Part model, mm, in its own coordinate system. A direction names the side the tool comes from. Round coordinates to 2 decimals unless told otherwise and drop trailing zeros. Write each loop counter-clockwise with the first axis right and the second up, starting at its lowest first coordinate (ties: lowest second). Pieces come first, ordered by that corner, then holes. Notation, with made-up numbers: M -16.5,19 L 34.5,19 A18 cw 34.5,47 Z; hole C 58.25,29 d6. An arc over 180 degrees is marked long. Use a Markdown table: item, result. Add a question column.
1) Drop flat-ended pins along their axis: P1, Ø6, axis at x = 1348.5, y = 740, coming from the -Z side; P2, Ø5, axis at x = 292.5, y = 429, coming from the +Z side; P3, Ø10, axis at y = 860, z = -823.5, coming from the +X side. Give the stop position or say it passes through.
2) Slice it at A-A on y = 587. Write the cut outline in (x, z), plus the area to 3 significant figures.
3) Which spindle directions (+Z, -Z, +X, -X, +Y, -Y) get a long thin tool onto all of the face, cutting with end or side? Do faces 4 (the face through (1266, 508, -129)), 5 (the face through (1270, 501, -758)), 6 (the face through (1016, 561, -307)). Say none if no direction does.
4) Slice it at B-B on x = 1042.5. Write the cut outline in (y, z).
5) Slice it at D-D on y = 353. Write the cut outline in (x, z).
6) Slice it at C-C on z = -487.5. Write the cut outline in (x, y).
7) Wall check: probe 1 along Y at (x, z) = (1159, -176); probe 2 along Z at (x, y) = (1097, 419); probe 3 along Z at (x, y) = (921, 594.5). Give the ranges that are in metal, low to high.
8) Two-plate mould, pull along Y, no slides. Class faces 1 (the face through (1524, 376, -258)), 2 (the face through (1274, 762, -258)), 3 (the face through (582, 254, -258)): released by +Y, released by -Y, zero draft, split by the parting line, or undercut.
```python
from build123d import *

# Parameters (mm, degrees)
SKETCH1_W           = 1016
SKETCH1_H           = 508
BOSS_EXTRUDE1_DEPTH = 254
BOSS_EXTRUDE2_DEPTH = 1016
BOSS_EXTRUDE3_DEPTH = 762
SKETCH2_W           = 254
SKETCH2_H           = 254
CUT_EXTRUDE3_DEPTH  = 508


with BuildPart() as part:
    # Sketch1 → Boss-Extrude1 (new body)
    with BuildSketch(Plane(origin=(0, 0, 0), x_dir=(1, 0, 0), z_dir=(0, 1, 0))):
        with Locations((508, 254)):
            Rectangle(SKETCH1_W, SKETCH1_H)
    extrude(amount=BOSS_EXTRUDE1_DEPTH)

    # Sketch1_3 → Boss-Extrude2 (add)
    with BuildSketch(Plane(origin=(0, 0, 0), x_dir=(1, 0, 0), z_dir=(0, 1, 0))):
        Polygon((0, 1016), (0, 508), (1016, 508), (1270, 508), (1270, 1016), align=None)
    extrude(amount=BOSS_EXTRUDE2_DEPTH)

    # Sketch1_4 → Boss-Extrude3 (add)
    with BuildSketch(Plane(origin=(0, 0, 0), x_dir=(1, 0, 0), z_dir=(0, 1, 0))):
        Polygon((1016, 508), (1270, 508), (1524, 508), (1524, 0), (1016, 0), align=None)
    extrude(amount=BOSS_EXTRUDE3_DEPTH)

    # Sketch2 → Cut-Extrude3 (cut)
    with BuildSketch(Plane.ZY.offset(-1016)):
        with Locations((-127, 381)):
            Rectangle(SKETCH2_W, SKETCH2_H)
    extrude(amount=-CUT_EXTRUDE3_DEPTH, mode=Mode.SUBTRACT)


solid = part.part
```
Entries:
| question | item | result |
|---|---|---|
| 1 | P1 | stops at z = -508 |
| 1 | P2 | stops at z = -508 |
| 1 | P3 | stops at x = 1270 |
| 2 | outline | M 0,-1016 L 1270,-1016 L 1270,-508 L 1524,-508 L 1524,0 L 1016,0 L 1016,-508 L 0,-508 Z |
| 2 | area | 903,000 mm^2 |
| 3 | face 4 | +Z, +X, -X |
| 3 | face 5 | -Z, +X, +Y, -Y |
| 3 | face 6 | +Z, -X, +Y |
| 4 | outline | M 0,-1016 L 1016,-1016 L 1016,-508 L 762,-508 L 762,0 L 508,0 L 508,-254 L 254,-254 L 254,0 L 0,0 Z |
| 5 | outline | M 0,-1016 L 1270,-1016 L 1270,-508 L 1524,-508 L 1524,-254 L 1016,-254 L 1016,-508 L 0,-508 Z |
| 6 | outline | M 0,0 L 1524,0 L 1524,762 L 1016,762 L 1016,254 L 0,254 Z |
| 7 | probe 1 | y = 0 to 254, 508 to 762 |
| 7 | probe 2 | z = -1016 to -254 |
| 7 | probe 3 | z = -1016 to -508 |
| 8 | face 1 | zero draft |
| 8 | face 2 | released by +Y |
| 8 | face 3 | undercut |
